The model under review builds one solid part; all positions refer to its coordinate system, in mm. A direction names the side the tool comes from. Round coordinates to 2 decimals unless told otherwise and drop trailing zeros. Answer as CSV lines item,"result".
from build123d import *

# Parameters (mm, degrees)
BOSS_EXTRUDE1_DEPTH = 1.5
SKETCH2_R           = 1.325
CUT_EXTRUDE1_DEPTH  = 2.5
SKETCH3_R           = 0.5
CUT_EXTRUDE2_DEPTH  = 2.5
LPATTERN1_COUNT     = 20
LPATTERN1_PITCH     = 2.54
SKETCH5_R           = 0.5
CUT_EXTRUDE4_DEPTH  = 2.5
SKETCH4_R           = 3
CUT_EXTRUDE3_DEPTH  = 0.1


with BuildPart() as part:
    # Sketch1 → Boss-Extrude1 (new body)
    with BuildSketch(Plane(origin=(0, 0, 0), x_dir=(1, 0, 0), z_dir=(0, 1, 0))):
        with BuildLine():
            Line((-28.75, 15), (28.75, 15))
            ThreePointArc((28.75, 15), (31.401650429, 13.901650429), (32.5, 11.25))
            Line((32.5, 11.25), (32.5, -11.25))
            ThreePointArc((32.5, -11.25), (31.401650429, -13.901650429), (28.75, -15))
            Line((28.75, -15), (-28.75, -15))
            ThreePointArc((-28.75, -15), (-31.401650429, -13.901650429), (-32.5, -11.25))
            Line((-32.5, -11.25), (-32.5, 11.25))
            ThreePointArc((-32.5, 11.25), (-31.401650429, 13.901650429), (-28.75, 15))
        make_face()
    extrude(amount=BOSS_EXTRUDE1_DEPTH)

    # Sketch2 → Cut-Extrude1 (cut, through all)
    with BuildSketch(Plane(origin=(0, 1.5, 0), x_dir=(1, 0, 0), z_dir=(0, 1, 0))):
        with Locations((-29.025, 11.525)):
            Circle(SKETCH2_R)
        with Locations((29.025, 11.525)):
            Circle(SKETCH2_R)
        with Locations((29.025, -11.525)):
            Circle(SKETCH2_R)
        with Locations((-29.025, -11.525)):
            Circle(SKETCH2_R)
    extrude(amount=-CUT_EXTRUDE1_DEPTH, mode=Mode.SUBTRACT)

    # Sketch3 → Cut-Extrude2 (cut, through all)
    with BuildSketch(Plane(origin=(0, 1.5, 0), x_dir=(1, 0, 0), z_dir=(0, 1, 0))):
        with Locations((-24.128, 13)):
            Circle(SKETCH3_R)
        with Locations((-24.128, 10.5)):
            Circle(SKETCH3_R)
    cut_extrude2 = extrude(amount=-CUT_EXTRUDE2_DEPTH, mode=Mode.SUBTRACT)

    # LPattern1: Cut-Extrude2 ×20
    with Locations(*[(i * LPATTERN1_PITCH, 0, 0) for i in range(1, LPATTERN1_COUNT)]):
        add(cut_extrude2, mode=Mode.SUBTRACT)

    # Sketch5 → Cut-Extrude4 (cut, through all)
    with BuildSketch(Plane(origin=(0, 1.5, 0), x_dir=(1, 0, 0), z_dir=(0, 1, 0))):
        with Locations((21.592, 5.5)):
            Circle(SKETCH5_R)
        with Locations((24.132, 5.5)):
            Circle(SKETCH5_R)
        with Locations((21.592, 8)):
            Circle(SKETCH5_R)
        with Locations((24.132, 8)):
            Circle(SKETCH5_R)
    extrude(amount=-CUT_EXTRUDE4_DEPTH, mode=Mode.SUBTRACT)

    # Sketch4 → Cut-Extrude3 (cut)
    with BuildSketch(Plane(origin=(0, 1.5, 0), x_dir=(1, 0, 0), z_dir=(0, 1, 0))):
        with Locations((-29.025, 11.525)):
            Circle(SKETCH4_R)
        with Locations((-29.025, -11.525)):
            Circle(SKETCH4_R)
        with Locations((29.025, -11.525)):
            Circle(SKETCH4_R)
        with Locations((29.025, 11.525)):
            Circle(SKETCH4_R)
        Polygon((-25.5, 14.3), (25.5, 14.3), (25.5, 9.2), (25.5, 4.2), (20.4, 4.2), (20.4, 9.2), (-25.5, 9.2), align=None)
    extrude(amount=-CUT_EXTRUDE3_DEPTH, mode=Mode.SUBTRACT)


solid = part.part
1. Tool access review of faces 1 (the face through (0, 0, 0)), 2 (the face through (30, 1.4, -10)): name each direction out of +Z, -Z, +X, -X, +Y, -Y from which nothing blocks a thin tool from reaching the whole face with its end or side.
Numbers:
face 1,"+Z, -Z, +X, -X, -Y"
face 2,"+Y"
2. Wall thickness on probe 1 along X at (y, z) = (1, -5.5); probe 2 along Z at (x, y) = (-11.5, 0.3); probe 3 along X at (y, z) = (1.1, 11.5): over which ranges is each line inside the solid? List them lowest first.
Numbers:
probe 1,"x = -32.5 to 21.09, 22.09 to 23.63, 24.63 to 32.5"
probe 2,"z = -15 to -13.49, -12.51 to -10.99, -10.01 to 15"
probe 3,"x = -32.49 to -30.35, -27.7 to 27.7, 30.35 to 32.49"
3. Take a section at A-A (y = 0.65). State how many separate pieces and enclosed holes the cut face has, plus the area to 3 significant figures.
Numbers:
separate pieces,"1"
enclosed holes,"48"
area,"1,880 mm²"
4. Clearance check with a flat-ended pin moving along its axis: pin 1 (1.8 mm diameter, centred on x = 28, z = 12.5, fed in from +Y). State where the tip first meets the part, or that it passes through.
Numbers:
pin 1,"stops at y = 1.4"
